```python
from build123d import *

# Parameters (mm, degrees)
F0_W     = 50.8
F0_H     = 31.75
F1_DEPTH = 38.1
F3_DEPTH = 31.75
F5_DEPTH = 25.4


with BuildPart() as f1:
    # F0 (on Front) → F1 (new body)
    with BuildSketch(Plane.XZ):
        with Locations((25.4, 15.875)):
            Rectangle(F0_W, F0_H)
    extrude(amount=F1_DEPTH)

    # F2 (on face) → F3 (cut)
    with BuildSketch(Plane.XY.offset(31.75)):
        with BuildLine():
            Line((50.8, -30.196967), (50.8, -7.903033))
            ThreePointArc((50.8, -7.903033), (39.653033, -19.05), (50.8, -30.196967))
        make_face()
    extrude(amount=-F3_DEPTH, mode=Mode.SUBTRACT)

    # F4 (on face) → F5 (cut)
    with BuildSketch(Plane(origin=(0, 0, 0), x_dir=(0, -1, 0), z_dir=(-1, 0, 0))):
        with BuildLine():
            Line((38.1, 31.75), (12.7, 31.75))
            ThreePointArc((12.7, 31.75), (20.139488, 13.789488), (38.1, 6.35))
            Line((38.1, 6.35), (38.1, 31.75))
        make_face()
    extrude(amount=-F5_DEPTH, mode=Mode.SUBTRACT)


solid = f1.part
```
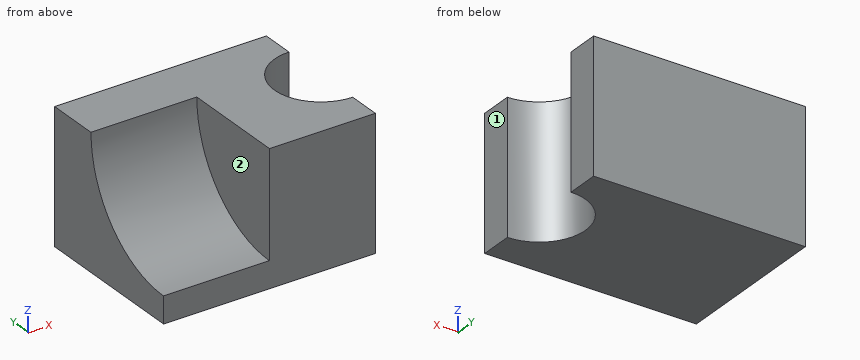
Read the model definition and answer for the solid it produces. Units are mm, in the model's axes. Face numbers are marked on the shaded views. A direction names the side the tool comes from. Round coordinates to 2 decimals unless told otherwise and drop trailing zeros. Write each loop counter-clockwise with the first axis right and the second up, starting at its lowest first coordinate (ties: lowest second). Pieces come first, ordered by that corner, then holes. Notation, with made-up numbers: (89.25, -2.5) -> (141.25, -2.5) arc R12 ccw to (141.25, 9.5) -> close; hole circle Ø4 at (71, 42). An arc over 180 degrees is marked (long way). Answer in a Markdown table with one row per item. Add a question column.
1) Find section A-A, the plane x = 41. Determine the outline of the cut face in (y, z), and give its area (3 significant figures).
2) Find section B-B, the plane z = 22. Determine the outline of the cut face in (x, y).
3) Find section C-C, the plane y = -19.5. Determine the outline of the cut face in (x, z), and give its area (3 significant figures).
4) Find section D-D, the plane x = 13.5. Determine the outline of the cut face in (y, z).
5) Which of the six approach directions +Z, -Z, +X, -X, +Y, -Y give full straight-line access (tool end or side, diameter ignored) to the marked faces 1 and 2?
6) Given P1, Ø2, axis at x = 19, y = -30.5, coming from the +Z side; P2, Ø1.5, axis at y = -34, z = 14.5, coming from the -X side, each flat-ended and moving along its own axis, determine where each tip first touches the part or whether it passes through.
7) Consider line 1 (Y direction, x = 43, z = 30); line 2 (X direction, y = -33, z = 28); line 3 (Z direction, x = 24, y = -24). Determine where each line is inside the solid, lowest interval first.
Findings below:
| question | item | result |
|---|---|---|
| 1 | outline | (-38.1, 0) -> (-24.36, 0) -> (-24.36, 31.75) -> (-38.1, 31.75) -> close; (-13.74, 0) -> (0, 0) -> (0, 31.75) -> (-13.74, 31.75) -> close |
| 1 | area | 872 mm² |
| 2 | outline | (0, -14.65) -> (25.4, -14.65) -> (25.4, -38.1) -> (50.8, -38.1) -> (50.8, -30.2) arc R11.15 cw to (50.8, -7.9) -> (50.8, 0) -> (0, 0) -> close |
| 3 | outline | (0, 0) -> (39.66, 0) -> (39.66, 31.75) -> (25.4, 31.75) -> (25.4, 14.45) -> (0, 14.45) -> close |
| 3 | area | 820 mm² |
| 4 | outline | (-38.1, 0) -> (0, 0) -> (0, 31.75) -> (-12.7, 31.75) arc R25.4 cw to (-38.1, 6.35) -> close |
| 5 | face 1 | +Z, -Z, +X, +Y, -Y |
| 5 | face 2 | +Z, -X, -Y |
| 6 | P1 | z = 7.85 |
| 6 | P2 | x = 25.4 |
| 7 | line 1 | -38.1 to -27.01, -11.09 to 0 |
| 7 | line 2 | 25.4 to 50.8 |
| 7 | line 3 | 0 to 10.62 |
